Answer from the drawing. Dimensions are ordinates in mm from the lowest x, y and z of the part. A direction names the side the tool comes from. Give positions to 0.01 mm unless a question says otherwise; leave off trailing zeros. Write each loop counter-clockwise with the first axis right and the second up, starting at its lowest first coordinate (ties: lowest second). Pieces come first, ordered by that corner, then holes.
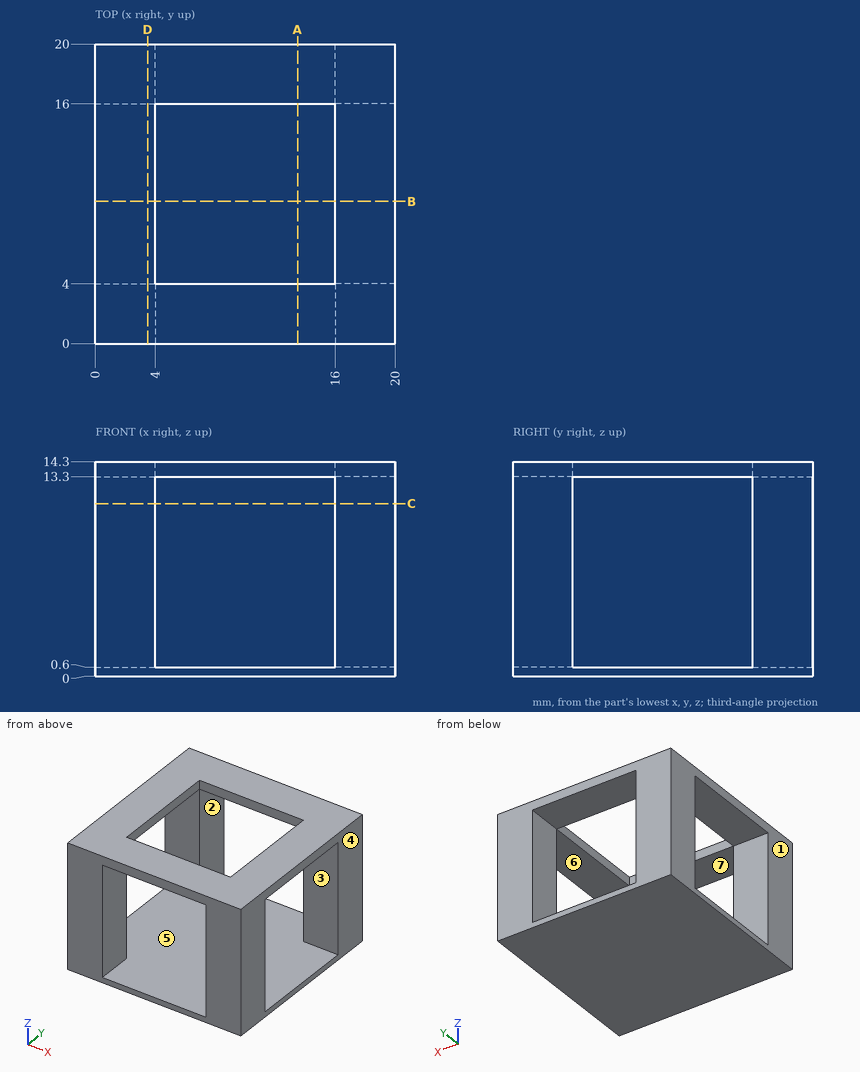
Item 1: Each of these flat-tipped pins is pushed along its axis until it touches: P1, Ø1, axis at x = 17.5, z = 2.5, coming from the -Y side; P2, Ø5, axis at y = 9, z = 10.5, coming from the +X side. Where does it stop, or does it pass through?
Conclusion:
P1: stops at y = 0
P2: passes through
Item 2: A cutting plane is placed at D-D, the plane x = 3.5. Give the vertices of the cut face in (y, z).
Conclusion:
outline: (0, 0) - (20, 0) - (20, 14.3) - (0, 14.3) - close; hole (4, 0.6) - (16, 0.6) - (16, 13.3) - (4, 13.3) - close
Item 3: A cutting plane is placed at A-A, the plane x = 13.5. Give the vertices of the cut face in (y, z).
Conclusion:
outline: (0, 0) - (20, 0) - (20, 0.6) - (0, 0.6) - close; (0, 13.3) - (4, 13.3) - (4, 14.3) - (0, 14.3) - close; (16, 13.3) - (20, 13.3) - (20, 14.3) - (16, 14.3) - close
Item 4: Determine the mould class of the marked faces 1, 2, 3 and 4 for opening direction X: pulls with the +X half, pulls with the -X half, needs draft (parallel to the pull), parting line crosses it, or undercut.
Conclusion:
face 1: pulls with the -X half
face 2: undercut
face 3: needs draft
face 4: pulls with the +X half
Item 5: Consider probe 1 along X at (y, z) = (3.75, 6.5); probe 2 along Z at (x, y) = (8.25, 1.75). Determine where each line is inside the solid, lowest interval first.
Conclusion:
probe 1: x = 0 to 4, 16 to 20
probe 2: z = 0 to 0.6, 13.3 to 14.3
Item 6: Which of the six approach directions +Z, -Z, +X, -X, +Y, -Y give full straight-line access (tool end or side, diameter ignored) to the marked faces 5, 6 and 7?
Conclusion:
face 5: none
face 6: +X, -X
face 7: +Y, -Y
Item 7: A cutting plane is placed at C-C, the plane z = 11.5. Give the vertices of the cut face in (x, y), plus the area to 3 significant figures.
Conclusion:
outline: (0, 0) - (4, 0) - (4, 4) - (0, 4) - close; (0, 16) - (4, 16) - (4, 20) - (0, 20) - close; (16, 0) - (20, 0) - (20, 4) - (16, 4) - close; (16, 16) - (20, 16) - (20, 20) - (16, 20) - close
area: 64.0 mm2
